```python
from build123d import *

# Parameters (mm, degrees)
BOSS_EXTRUDE1_DEPTH = 2


with BuildPart() as part:
    # Sketch1 → Boss-Extrude1 (new body)
    with BuildSketch(Plane(origin=(0, 0, 0), x_dir=(0, 0, -1), z_dir=(1, 0, 0))):
        with BuildLine():
            Line((-2, -2.5), (1.5, -2.5))
            Line((1.5, -2.5), (1.5, 0.193510405))
            Line((1.5, 0.193510405), (1.5, 0.544384676))
            Line((1.5, 0.544384676), (1.5, 1.260642871))
            Line((1.5, 1.260642871), (-0.25, 2.5))
            ThreePointArc((-0.25, 2.5), (-0.575, 3.379967104), (0.243957235, 2.9225))
            Line((0.243957235, 2.9225), (1.5, 2.010642871))
            Line((1.5, 2.010642871), (1.5, 3))
            ThreePointArc((1.5, 3), (-0.25, 4.75), (-2, 3))
            Line((-2, 3), (-2, -2.5))
        make_face()
    extrude(amount=BOSS_EXTRUDE1_DEPTH)


solid = part.part
```
Could you check a few things on this model? Use its own coordinates, in mm. A direction names the side the tool comes from. Coordinates: 2 decimals unless noted, no trailing zeros. Write each loop counter-clockwise with the first axis right and the second up, starting at its lowest first coordinate (ties: lowest second). Pieces come first, ordered by that corner, then holes. Notation, with made-up numbers: (-2.5, 69.25) - (3.5, 69.25) arc R6 ccw to (3.5, 74.25) - close; hole circle Ø3 at (61, -32.5). An arc over 180 degrees is marked (long way). Use a Markdown table: item, result.
Q1. I'm going to push flat-ended pins straight in: pin 1 Ø0.9 at (y, z) = (3, 0.25) entering from -X; pin 2 Ø1 at (y, z) = (3, 0) entering from -X; pin 3 Ø1 at (x, z) = (1.5, 1.5) entering from +Y. Where does each tip first touch, or does it pass through?
Geometry check:
| item | result |
|---|---|
| pin 1 | passes through |
| pin 2 | stops at x = 0 |
| pin 3 | stops at y = 4.58 |
Q2. Imagine slicing it at D-D (z = 1.6). List the corners of the cut face in (x, y) for me, and give its area (3 significant figures).
Geometry check:
| item | result |
|---|---|
| outline | (0, -2.5) - (2, -2.5) - (2, 4.11) - (0, 4.11) - close |
| area | 13.2 mm2 |
Q3. Which directions (+Z, -Z, +X, -X, +Y, -Y) give clear straight access to the entire face, cutting with the end or side of a thin tool? Please do faces 4 (the flat face through (0.986, 2.473, -0.863)), 5 (the flat face through (0, 1, 0)).
Geometry check:
| item | result |
|---|---|
| face 4 | +X, -X |
| face 5 | +Z, -Z, -X, +Y, -Y |
Q4. Imagine slicing it at B-B (x = 0.4). List the corners of the cut face in (y, z) for me.
Geometry check:
| item | result |
|---|---|
| outline | (-2.5, -1.5) - (1.26, -1.5) - (2.5, 0.25) arc R0.5 cw (long way) to (2.92, -0.24) - (2.01, -1.5) - (3, -1.5) arc R1.75 ccw to (3, 2) - (-2.5, 2) - close |
Q5. Imagine slicing it at A-A (z = -0.05). List the corners of the cut face in (x, y) for me, and give its area (3 significant figures).
Geometry check:
| item | result |
|---|---|
| outline | (0, -2.5) - (2, -2.5) - (2, 2.29) - (0, 2.29) - close; (0, 3.4) - (2, 3.4) - (2, 4.72) - (0, 4.72) - close |
| area | 12.2 mm2 |
Q6. Imagine slicing it at C-C (z = 1.1). List the corners of the cut face in (x, y) for me, and give its area (3 significant figures).
Geometry check:
| item | result |
|---|---|
| outline | (0, -2.5) - (2, -2.5) - (2, 4.53) - (0, 4.53) - close |
| area | 14.1 mm2 |
Q7. Please list where these lines run through material, in increasing order: L1, parallel to Z at x = 1.15, y = 3; L2, parallel to Y at x = 1.3, z = -0.45; L3, parallel to Y at x = 1.8, z = -1.2.
Geometry check:
| item | result |
|---|---|
| L1 | z = -1.5 to -0.25, 0.75 to 2 |
| L2 | y = -2.5 to 2, 2.77 to 4.6 |
| L3 | y = -2.5 to 1.47, 2.23 to 3.98 |
Q8. Thinking about a two-plate mould opening in Y: for faces 1 (the flat face through (1, -1, -1.5)), 2 (the flat face through (1, 1.9, -0.6)), 3 (the cylindrical face through (0.99, 4.75, 0.21)), which applies, +Y half, -Y half, draft (parallel to the pull), parting line (faces both ways), or undercut?
Geometry check:
| item | result |
|---|---|
| face 1 | draft |
| face 2 | undercut |
| face 3 | +Y half |
